For this review, take the finished solid that the model builds, in its own axes (mm). A direction names the side the tool comes from. Round coordinates to 2 decimals unless told otherwise and drop trailing zeros. Write each loop counter-clockwise with the first axis right and the second up, starting at its lowest first coordinate (ties: lowest second). Pieces come first, ordered by that corner, then holes. Notation, with made-up numbers: (31.5, -19) -> (54.5, -19) arc R31 ccw to (54.5, 8) -> close; hole circle Ø3 at (-32.5, 26.25). An arc over 180 degrees is marked (long way). Answer as CSV lines item,"result". Start each with the question number.
Item 1: Take a section at A-A on z = 0. Give the boundary of the cut face in (x, y).
Item 2: Take a section at B-B on x = 0. Give the boundary of the cut face in (y, z), then the cut area to 3 significant figures.
Item 3: Wall thickness on probe 1 along X at (y, z) = (-0.3, 0); probe 2 along X at (y, z) = (-4.4, 0); probe 3 along Z at (x, y) = (-1, -5): over which ranges is each line inside the solid? List them lowest first. Write a range as from..to.
Item 4: Take a section at D-D on z = 37. Give the boundary of the cut face in (x, y).
Item 5: Take a section at C-C on y = -3.5. Give the boundary of the cut face in (x, z).
Item 6: For pin 1 Ø6 at (x, z) = (-0.5, -16.5) entering from +Y; pin 2 Ø1 at (x, y) = (22, -2) entering from -Z; pin 3 Ø7 at (x, z) = (-37, 0) entering from -Y; pin 4 Ø5 at (x, z) = (0, -37) entering from +Y, all flat-tipped, find the tip position at first contact; note any pin that passes through.
Item 7: Machinability: for faces 1 (the cylindrical face through (0.358, -0.035, -39.727)), 2 (the cylindrical face through (20.633, -3.979, 15.821)), which of the approach directions +Z, -Z, +X, -X, +Y, -Y give a long, thin tool a straight path to every point of the face, cutting with its end or side? Answer none if there is none.
Item 8: Mouldability with a two-part tool opening along X and no side actions: class faces 3 (the flat face through (-5, -2.5, -18)), 4 (the cylindrical face through (33.727, -0.035, 25.861)), 5 (the flat face through (22.24, -2.5, 21.84)) as +X half, -X half, draft (parallel to the pull), parting line (faces both ways), or undercut.
```python
from build123d import *

# Parameters (mm, degrees)
M5_CLEARANCE_HOLE1_D = 5.5
CIRPATTERN1_COUNT    = 4


with BuildPart() as part:
    # Sketch1 → Revolve1 (revolve)
    with BuildSketch(Plane.XY):
        Polygon((-18, 2.5), (-42.5, 2.5), (-42.5, -2.5), (-31, -2.5), (-31, -5.5), (-26, -5.5), (-26, -2.5), (-18, -2.5), align=None)
    revolve(axis=Axis((0, 0, 0), (0, -1, 0)))

    # M5 Clearance Hole1 (through all)
    with Locations(Plane(origin=(37, 2.5, 0), x_dir=(0, 0, 1), z_dir=(0, 1, 0))):
        with Locations((0, 0)):
            m5_clearance_hole1 = Hole(M5_CLEARANCE_HOLE1_D / 2)

    # CirPattern1: M5 Clearance Hole1 ×4 about axis
    cirpattern1_axis = Axis((0, 0, 0), (0, 1, 0))
    for i in range(1, CIRPATTERN1_COUNT):
        add(m5_clearance_hole1.rotate(cirpattern1_axis, i * 360 / CIRPATTERN1_COUNT), mode=Mode.SUBTRACT)


solid = part.part
```
Output values:
1,outline,"(-42.5, -2.5) -> (-39.75, -2.5) -> (-39.75, 2.5) -> (-42.5, 2.5) -> close; (-34.25, -2.5) -> (-31, -2.5) -> (-31, -5.5) -> (-26, -5.5) -> (-26, -2.5) -> (-18, -2.5) -> (-18, 2.5) -> (-34.25, 2.5) -> close; (18, -2.5) -> (26, -2.5) -> (26, -5.5) -> (31, -5.5) -> (31, -2.5) -> (34.25, -2.5) -> (34.25, 2.5) -> (18, 2.5) -> close; (39.75, -2.5) -> (42.5, -2.5) -> (42.5, 2.5) -> (39.75, 2.5) -> close"
2,outline,"(-5.5, -31) -> (-2.5, -31) -> (-2.5, -34.25) -> (2.5, -34.25) -> (2.5, -18) -> (-2.5, -18) -> (-2.5, -26) -> (-5.5, -26) -> close; (-5.5, 26) -> (-2.5, 26) -> (-2.5, 18) -> (2.5, 18) -> (2.5, 34.25) -> (-2.5, 34.25) -> (-2.5, 31) -> (-5.5, 31) -> close; (-2.5, -42.5) -> (2.5, -42.5) -> (2.5, -39.75) -> (-2.5, -39.75) -> close; (-2.5, 39.75) -> (2.5, 39.75) -> (2.5, 42.5) -> (-2.5, 42.5) -> close"
2,area,"220 mm^2"
3,probe 1,"x = -42.5..-39.75, -34.25..-18, 18..34.25, 39.75..42.5"
3,probe 2,"x = -31..-26, 26..31"
3,probe 3,"z = -30.98..-25.98, 25.98..30.98"
4,outline,"(-20.91, -2.5) -> (-2.75, -2.5) -> (-2.75, 2.5) -> (-20.91, 2.5) -> close; (2.75, -2.5) -> (20.91, -2.5) -> (20.91, 2.5) -> (2.75, 2.5) -> close"
5,outline,"circle Ø62 at (0, 0); hole circle Ø52 at (0, 0)"
6,pin 1,"stops at y = 2.5"
6,pin 2,"stops at z = -36.66"
6,pin 3,"stops at y = -2.5"
6,pin 4,"passes through"
7,face 1,"+Y, -Y"
7,face 2,"-Y"
8,face 3,"undercut"
8,face 4,"parting line"
8,face 5,"draft"
